```python
from build123d import *

# Parameters (mm, degrees)
SKETCH1_R           = 15.875
BOSS_EXTRUDE1_DEPTH = 82.55


with BuildPart() as part:
    # Sketch1 → Boss-Extrude1 (new, symmetric)
    with BuildSketch(Plane.XY):
        Circle(SKETCH1_R)
        with BuildLine():
            Line((-1.5, 5.291502622), (-1.5, 10.291502622))
            Line((-1.5, 10.291502622), (1.5, 10.291502622))
            Line((1.5, 10.291502622), (1.5, 5.291502622))
            ThreePointArc((1.5, 5.291502622), (2.75, 4.763139721), (3.832575695, 3.944789417))
            Line((3.832575695, 3.944789417), (8.162702714, 6.444789417))
            Line((8.162702714, 6.444789417), (9.662702714, 3.846713205))
            Line((9.662702714, 3.846713205), (5.332575695, 1.346713205))
            ThreePointArc((5.332575695, 1.346713205), (5.5, 0), (5.332575695, -1.346713205))
            Line((5.332575695, -1.346713205), (9.662702714, -3.846713205))
            Line((9.662702714, -3.846713205), (8.162702714, -6.444789417))
            Line((8.162702714, -6.444789417), (3.832575695, -3.944789417))
            ThreePointArc((3.832575695, -3.944789417), (2.75, -4.763139721), (1.5, -5.291502622))
            Line((1.5, -5.291502622), (1.5, -10.291502622))
            Line((1.5, -10.291502622), (-1.5, -10.291502622))
            Line((-1.5, -10.291502622), (-1.5, -5.291502622))
            ThreePointArc((-1.5, -5.291502622), (-2.75, -4.763139721), (-3.832575695, -3.944789417))
            Line((-3.832575695, -3.944789417), (-8.162702714, -6.444789417))
            Line((-8.162702714, -6.444789417), (-9.662702714, -3.846713205))
            Line((-9.662702714, -3.846713205), (-5.332575695, -1.346713205))
            ThreePointArc((-5.332575695, -1.346713205), (-5.5, 0), (-5.332575695, 1.346713205))
            Line((-5.332575695, 1.346713205), (-9.662702714, 3.846713205))
            Line((-9.662702714, 3.846713205), (-8.162702714, 6.444789417))
            Line((-8.162702714, 6.444789417), (-3.832575695, 3.944789417))
            ThreePointArc((-3.832575695, 3.944789417), (-2.75, 4.763139721), (-1.5, 5.291502622))
        make_face(mode=Mode.SUBTRACT)
    extrude(amount=BOSS_EXTRUDE1_DEPTH, both=True)


solid = part.part
```
Verification items for the finished model (mm, model axes). A direction names the side the tool comes from. Round coordinates to 2 decimals unless told otherwise and drop trailing zeros. Order: outer loops, then holes, each group sorted by start corner. A loop starts at its lowest first (then second) coordinate and runs counter-clockwise, first axis right, second up.
1) Draft check along X on faces 1 (the flat face through (7, 0, 82.55)), 2 (the flat face through (-8.92, 5.13, 1.16)), 3 (the flat face through (-6.028, 5.212, 1.156)). Enter one of: +X half, -X half, draft (parallel to the pull), parting line (faces both ways), or undercut.
Geometry says:
face 1: draft
face 2: undercut
face 3: undercut
2) Cross-section at C-C, the plane y = -8.5. Record the cut outline in (x, z), plus the area to 3 significant figures.
Geometry says:
outline: (-13.41, -82.55) - (-1.5, -82.55) - (-1.5, 82.55) - (-13.41, 82.55) - close; (1.5, -82.55) - (13.41, -82.55) - (13.41, 82.55) - (1.5, 82.55) - close
area: 3,930 mm2
3) Depth check by flat-ended pin: pin 1 (8 mm diameter, centred on y = -6, z = 35, fed in from -X); pin 2 (4 mm diameter, centred on y = 9, z = -4, fed in from -X); pin 3 (4 mm diameter, centred on y = 7.5, z = -12, fed in from -X). Enter the tip coordinate at first touch or a pass-through.
Geometry says:
pin 1: stops at x = -15.75
pin 2: stops at x = -14.25
pin 3: stops at x = -14.89
4) Cross-section at D-D, the plane x = 13. Record the cut outline in (y, z).
Geometry says:
outline: (-9.11, -82.55) - (9.11, -82.55) - (9.11, 82.55) - (-9.11, 82.55) - close
5) Tool access check on faces 4 (the flat face through (-1.5, 8, 1)), 5 (the flat face through (7, 0, -82.55)). Record the directions out of +Z, -Z, +X, -X, +Y, -Y that give a thin tool (end or side, any length) a straight path to the whole face; none if there is none.
Geometry says:
face 4: +Z, -Z
face 5: -Z, +X, -X, +Y, -Y
6) Material ranges on line 1 (Y direction, x = -7.5, z = 14.5); line 2 (Y direction, x = -0.5, z = -12.5); line 3 (Y direction, x = -7, z = 5), recorded low to high.
Geometry says:
line 1: y = -13.99 to -6.06, -2.6 to 2.6, 6.06 to 13.99
line 2: y = -15.87 to -10.29, 10.29 to 15.87
line 3: y = -14.25 to -5.77, -2.31 to 2.31, 5.77 to 14.25
